The figure shows three views and two pictorial views of one solid part (mm, origin at its lowest corner). Answer the questions. A direction names the side the tool comes from. Round coordinates to 2 decimals unless told otherwise and drop trailing zeros. Order: outer loops, then holes, each group sorted by start corner. A loop starts at its lowest first (then second) coordinate and runs counter-clockwise, first axis right, second up. Notation, with made-up numbers: (60.25, 47) - (106.25, 47) arc R10 ccw to (106.25, 53) - close; hole circle Ø2 at (-0.5, 59). An arc over 180 degrees is marked (long way). Answer as a JSON object with one key per item and string values. Group by question number.
Q1. Consider line 1 (Z direction, x = 17.75, y = 12); line 2 (X direction, y = 13, z = 3.5); line 3 (X direction, y = 14.5, z = 3.75). Determine where each line is inside the solid, lowest interval first.
Q2. A cutting plane is placed at A-A on z = 2. Determine the outline of the cut face in (x, y), and give its area (3 significant figures).
Q3. A cutting plane is placed at B-B on z = 5.75. Determine the outline of the cut face in (x, y).
Q4. A tool of negligible diameter and unlimited length cuts with its end or side. For the marked faces 1, 2 and 3, from which of +Z, -Z, +X, -X, +Y, -Y can it reach the whole face along a straight path? Write none if from no direction.
Q5. A cutting plane is placed at D-D on x = 9. Determine the outline of the cut face in (y, z).
Q6. Given pin 1 Ø14 at (x, y) = (17, 6.5) entering from +Z; pin 2 Ø3 at (x, z) = (17.5, 1) entering from -Y; pin 3 Ø3 at (x, y) = (4.5, 19) entering from +Z; pin 4 Ø2 at (x, z) = (18.5, 6.5) entering from -Y, each flat-ended and moving along its own axis, determine where each tip first touches the part or whether it passes through.
Q7. A cutting plane is placed at C-C on y = 10.75. Determine the outline of the cut face in (x, z).
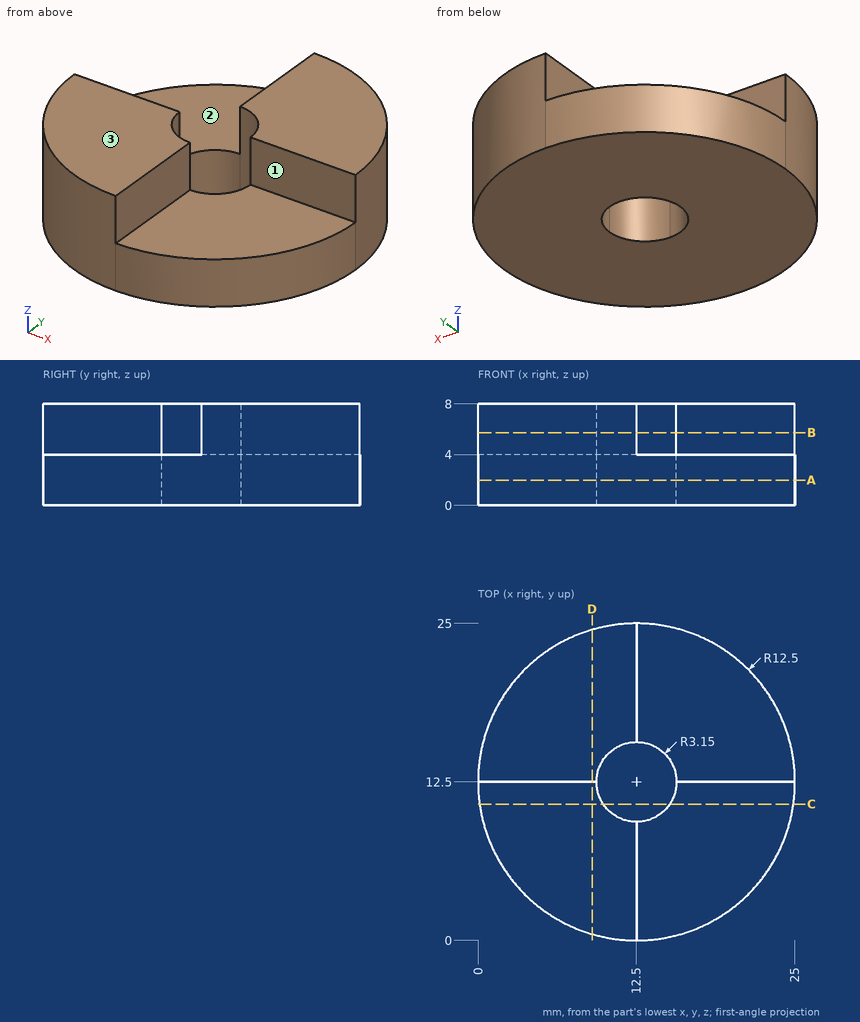
Result set:
{
 "1": {"line 1": "z = 0 to 4", "line 2": "x = 0.01 to 9.39, 15.61 to 24.99", "line 3": "x = 0.16 to 10.07, 14.93 to 24.84"},
 "2": {"outline": "(0, 12.5) arc R12.5 ccw to (12.5, 0) arc R12.5 ccw to (25, 12.5) arc R12.5 ccw to (12.5, 25) arc R12.5 ccw to start; hole (9.35, 12.5) arc R3.15 ccw to (12.5, 9.35) arc R3.15 ccw to (15.65, 12.5) arc R3.15 ccw to (12.5, 15.65) arc R3.15 ccw to start", "area": "460 mm²"},
 "3": {"outline": "(0, 12.5) arc R12.5 ccw to (12.5, 0) - (12.5, 9.35) arc R3.15 cw to (9.35, 12.5) - close; (12.5, 15.65) arc R3.15 cw to (15.65, 12.5) - (25, 12.5) arc R12.5 ccw to (12.5, 25) - close"},
 "4": {"face 1": "+Z, +X, -Y", "face 2": "+Z, -X, +Y", "face 3": "+Z, +X, -X, +Y, -Y"},
 "5": {"outline": "(0.5, 0) - (24.5, 0) - (24.5, 4) - (12.5, 4) - (12.5, 8) - (0.5, 8) - close"},
 "6": {"pin 1": "stops at z = 8", "pin 2": "stops at y = 0.5", "pin 3": "stops at z = 4", "pin 4": "stops at y = 12.5"},
 "7": {"outline": "(0.12, 0) - (9.88, 0) - (9.88, 8) - (0.12, 8) - close; (15.12, 0) - (24.88, 0) - (24.88, 4) - (15.12, 4) - close"}
}
